Model file for the job. Use its own axes, mm. A direction names the side the tool comes from. Give positions to 0.01 mm unless a question says otherwise; leave off trailing zeros. Order: outer loops, then holes, each group sorted by start corner. A loop starts at its lowest first (then second) coordinate and runs counter-clockwise, first axis right, second up. Notation, with made-up numbers: M 61,21 L 71,21 A16 ccw 71,33 Z; hole C 72,4.5 d6. An arc over 180 degrees is marked long. Return JSON: item names as keys, results as strings. Group by question number.
1. Slice it at A-A on y = 0. List the corners of the cut face in (x, z), then the cut area to 3 significant figures.
2. Slice it at D-D on y = 31. List the corners of the cut face in (x, z), then the cut area to 3 significant figures.
3. Slice it at C-C on x = 233. List the corners of the cut face in (y, z), then the cut area to 3 significant figures.
4. Slice it at B-B on z = 2.5. List the corners of the cut face in (x, y), then the cut area to 3 significant figures.
5. Two-plate mould, pull along X, no slides. Class faces 1 (the face through (360.753, 12.465, 3.451)), 2 (the face through (354.032, -1.075, 3.451)), 3 (the face through (178.218, -1, 3)): released by +X, released by -X, zero draft, split by the parting line, or undercut.
6. 3-axis set-ups, long thin cutter, end or side, ignore diameter. For faces 4 (the face through (208.218, 35, 3)), 5 (the face through (208.218, -35, 3)), 6 (the face through (193, -60, 3)): which of +Z, -Z, +X, -X, +Y, -Y reach the whole face in a straight line?
7. Wall check: probe 1 along X at (y, z) = (0, 1.5); probe 2 along Y at (x, z) = (291, 5.25); probe 3 along X at (y, z) = (-24.5, 5.75). Give the ranges that are in metal, low to high. Write a range as [from, to].
8. Pin check, flat tips, straight feed: pin 1 (6.5 mm diameter, centred on x = 355.72, y = 0, fed in from -Z); pin 2 (3.5 mm diameter, centred on y = 44.5, z = 4.5, fed in from +X). Stop position of each tip, or through.
Autodesk Inventor part; units mm, degrees
ref_plane "YZ Plane" through (0, 0, 0) normal (1, 0, 0) x (0, 1, 0)
ref_plane "XZ Plane" through (0, 0, 0) normal (0, 1, 0) x (-1, 0, 0)
ref_plane "XY Plane" through (0, 0, 0) normal (0, 0, 1) x (1, 0, 0)
sketch "Sketch1" plane through (0, 0, 0) normal (0, 0, 1) x (1, 0, 0)
  line L0 (100, -75) -> (100, -15)
  line L1 (100, 75) -> (-100, 75)
  line L2 (-100, 75) -> (-100, -75)
  line L3 (-100, -75) -> (100, -75)
  arc A0 (-85, -15) -> (-85, 15) centre (-85, 0) ccw
  line L4 (-85, 15) -> (-85, 60)
  line L5 (-85, 60) -> (85, 60)
  line L6 (85, -15) -> (85, -60)
  line L7 (85, -60) -> (-85, -60)
  line L8 (-85, -60) -> (-85, -15)
  line L9 (183.2183, 60) -> (203.2183, 60)
  line L10 (203.2183, -60) -> (183.2183, -60)
  line L11 (178.2183, -55) -> (178.2183, 55)
  line L12 (208.2183, 0) -> (358.2183, 0) construction
  line L13 (208.2183, 15) -> (358.2183, 15)
  line L14 (208.2183, -15) -> (358.2183, -15)
  line L15 (363.2183, -10) -> (363.2183, 10)
  line L16 (208.2183, 55) -> (208.2183, 15)
  line L17 (208.2183, -15) -> (208.2183, -55)
  line L18 (85, 60) -> (85, 15)
  line L19 (85, 15) -> (100, 15)
  line L20 (100, 15) -> (100, 75)
  line L21 (100, -15) -> (85, -15)
  line L22 (358.2183, -15) -> (363.2183, -10)
  line L23 (363.2183, 10) -> (358.2183, 15)
  line L24 (178.2183, 55) -> (183.2183, 60)
  line L25 (203.2183, 60) -> (208.2183, 55)
  line L26 (208.2183, -55) -> (203.2183, -60)
  line L27 (183.2183, -60) -> (178.2183, -55)
  point P0 (0, 0)
  point P1 (178.2183, 60)
  point P2 (208.2183, -60)
  point P3 (208.2183, 60)
  point P4 (178.2183, -60)
  point P5 (363.2183, 15)
  point P6 (363.2183, -15)
  point P7 (1.2343, 60)
  point P8 (-28.7657, -60)
  point P9 (-3.7657, -60)
  point P10 (-23.7657, -60)
  point P11 (-23.7657, 60)
  point P12 (-3.7657, 60)
  dimension "d0" = 30
  dimension "d1" = 150
  dimension "d2" = 15
  dimension "d3" = 15
  dimension "d6" = 185
  dimension "d7" = 30
  dimension "d8" = 45
  dimension "d9" = 5
  dimension "d10" = 5
  dimension "d11" = 5
  dimension "d12" = 5
  dimension "d13" = 5
  dimension "d14" = 5
  dimension "d15" = 5
  dimension "d16" = 5
  dimension "d17" = 5
  dimension "d18" = 5
  dimension "d19" = 5
  dimension "d20" = 5
extrude "Extrusion1" add sketch "Sketch1" along normal blind 7 contours L9 L25 L16 L13 L23 L15 L22 L14 L17 L26 L10 L27 L11 L24
sketch "Sketch2" plane through (0, 0, 7) normal (0, 0, 1) x (1, 0, 0)
  line L0 (363.2183, -10) -> (363.2183, 10)
  point P0 (0, 0)
  point P1 (355.7183, 0)
  dimension "d21" = 7.5
hole "Hole1" at (355.7183, 0, 7) direction (0, 0, -1) diameter 4 end through all
equation "\"d1\" = lPiston"
equation "\"lPiston\" = 150"
properties part number "Piston" material "MDF Medium Density Fiberboard"
Result:
{
 "1": {"outline": "M 178.22,0 L 353.72,0 L 353.72,7 L 178.22,7 Z; M 357.72,0 L 363.22,0 L 363.22,7 L 357.72,7 Z", "area": "1,270 mm2"},
 "2": {"outline": "M 178.22,0 L 208.22,0 L 208.22,7 L 178.22,7 Z", "area": "210 mm2"},
 "3": {"outline": "M -15,0 L 15,0 L 15,7 L -15,7 Z", "area": "210 mm2"},
 "4": {"outline": "M 178.22,-55 L 183.22,-60 L 203.22,-60 L 208.22,-55 L 208.22,-15 L 358.22,-15 L 363.22,-10 L 363.22,10 L 358.22,15 L 208.22,15 L 208.22,55 L 203.22,60 L 183.22,60 L 178.22,55 Z; hole C 355.72,0 d4", "area": "8,160 mm2"},
 "5": {"face 1": "released by +X", "face 2": "undercut", "face 3": "released by -X"},
 "6": {"face 4": "+Z, -Z, +X, +Y", "face 5": "+Z, -Z, +X, -Y", "face 6": "+Z, -Z, +X, -X, -Y"},
 "7": {"probe 1": "x = [178.22, 353.72], [357.72, 363.22]", "probe 2": "y = [-15, 15]", "probe 3": "x = [178.22, 208.22]"},
 "8": {"pin 1": "stops at z = 0", "pin 2": "stops at x = 208.22"}
}
